Geometry: final body of the model. Coordinates: model frame, mm. Face numbers are marked on the shaded views. A direction names the side the tool comes from. Give positions to 0.01 mm unless a question says otherwise; leave off trailing zeros. Loops run counter-clockwise (first coordinate to the right, second up) from the corner with the lowest first, then second, coordinate; pieces in that order, holes last. Notation, with made-up numbers: (-14.5, 24.5) -> (-6.5, 24.5) arc R3 cw to (-6.5, 28.5) -> close; hole circle Ø5 at (35.5, 80). An arc over 180 degrees is marked (long way). One line per question, with ' | ' between items. Start each with the question number.
Item 1: Section A-A on y = 12.75. Return loops of the section in (x, z).
Item 2: Section B-B on x = -1.3. Return loops of the section in (y, z).
Item 3: Set-up query: the marked faces 1, 2 and 3. Return all of +Z, -Z, +X, -X, +Y, -Y with unobstructed straight access to the full face (end or side cutting, diameter ignored); none if empty.
Item 4: Section D-D on y = 7.25. Return loops of the section in (x, z), then the cut area to 3 significant figures.
Item 5: Mould query, pull axis Z, two halves, no side actions, for the marked faces 4, 5, 6 and 7. Classes: released by +Z, released by -Z, zero draft, split by the parting line, or undercut.
Item 6: Pin query (flat end, axial travel): P1, Ø1.8, axis at x = -0.5, z = 3.5, coming from the -Y side; P2, Ø1.2, axis at y = 4, z = 0, coming from the -X side; P3, Ø3, axis at y = 3.5, z = 1, coming from the +X side. Return the tip coordinate at first contact, or that it passes through.
Item 7: Material intervals for line 1 along Z through (x, y) = (-0.15, 14.5); line 2 along Y through (x, z) = (-2.3, -1.25); line 3 along Z through (x, y) = (-2.05, 13.25), sorted ascending. Write a range as [from, to].
Item 8: Section C-C on z = -0.5. Return loops of the section in (x, y), then the cut area to 3 significant figures.
from build123d import *

# Parameters (mm, degrees)
SKETCH1_W           = 1.506666666
SKETCH1_H           = 1.506666666
BOSS_EXTRUDE1_DEPTH = 15
SKETCH2_R           = 0.753333333
BOSS_EXTRUDE2_DEPTH = 1.666666667
SKETCH3_W           = 5.16
SKETCH3_H           = 1.666666667
SKETCH3_H_2         = 5.16
SKETCH3_W_2         = 1.506666666
SKETCH3_H_3         = 1.506666666
BOSS_EXTRUDE3_DEPTH = 2.5
SKETCH3_3_W         = 5.16
SKETCH3_3_H         = 1.666666667
BOSS_EXTRUDE4_DEPTH = 2.5


with BuildPart() as part:
    # Sketch1 → Boss-Extrude1 (new body)
    with BuildSketch(Plane(origin=(0, 0, 0), x_dir=(1, 0, 0), z_dir=(0, 1, 0))):
        Rectangle(SKETCH1_W, SKETCH1_H)
    extrude(amount=BOSS_EXTRUDE1_DEPTH)

    # Sketch2 → Boss-Extrude2 (add)
    with BuildSketch(Plane.XZ):
        with Locations(Location((0, 0, 0), (0, 0, 270))):
            Circle(SKETCH2_R)
    extrude(amount=BOSS_EXTRUDE2_DEPTH)

    # Sketch3 → Boss-Extrude3 (add)
    # profile 1 of 4: a face of its own
    with BuildSketch(Plane(origin=(0, 15, 0), x_dir=(1, 0, 0), z_dir=(0, 1, 0))):
        with Locations((0, 3.413333334)):
            Rectangle(SKETCH3_W, SKETCH3_H)
    # profile 2 of 4: a face of its own
    with BuildSketch(Plane(origin=(0, 15, 0), x_dir=(1, 0, 0), z_dir=(0, 1, 0))):
        Rectangle(SKETCH3_W, SKETCH3_H_2)
        Rectangle(SKETCH3_W_2, SKETCH3_H_3, mode=Mode.SUBTRACT)
    # profile 3 of 4: a face of its own
    with BuildSketch(Plane(origin=(0, 15, 0), x_dir=(1, 0, 0), z_dir=(0, 1, 0))):
        with Locations((0, -3.413333334)):
            Rectangle(SKETCH3_W, SKETCH3_H)
    # profile 4 of 4: a face of its own
    with BuildSketch(Plane(origin=(0, 15, 0), x_dir=(1, 0, 0), z_dir=(0, 1, 0))):
        Rectangle(SKETCH3_W_2, SKETCH3_H_3)
    extrude(amount=BOSS_EXTRUDE3_DEPTH)

    # Sketch3_3 → Boss-Extrude4 (add)
    with BuildSketch(Plane(origin=(0, 15, 0), x_dir=(1, 0, 0), z_dir=(0, 1, 0))):
        with Locations((0, 3.413333334)):
            Rectangle(SKETCH3_3_W, SKETCH3_3_H)
        with Locations((0, -3.413333334)):
            Rectangle(SKETCH3_3_W, SKETCH3_3_H)
    extrude(amount=-BOSS_EXTRUDE4_DEPTH)


solid = part.part
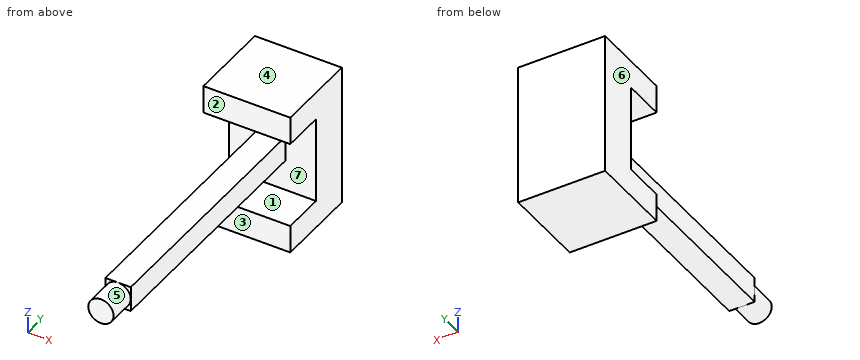
Result sheet:
1) outline: (-2.58, -4.25) -> (2.58, -4.25) -> (2.58, -2.58) -> (-2.58, -2.58) -> close; (-2.58, 2.58) -> (2.58, 2.58) -> (2.58, 4.25) -> (-2.58, 4.25) -> close; (-0.75, -0.75) -> (0.75, -0.75) -> (0.75, 0.75) -> (-0.75, 0.75) -> close
2) outline: (12.5, -4.25) -> (17.5, -4.25) -> (17.5, 4.25) -> (12.5, 4.25) -> (12.5, 2.58) -> (15, 2.58) -> (15, -2.58) -> (12.5, -2.58) -> close
3) face 1: +X, -X, -Y | face 2: +Z, +X, -X, -Y | face 3: -Z, +X, -X, -Y
4) outline: (-0.75, -0.75) -> (0.75, -0.75) -> (0.75, 0.75) -> (-0.75, 0.75) -> close | area: 2.27 mm²
5) face 4: released by +Z | face 5: split by the parting line | face 6: zero draft | face 7: undercut
6) P1: stops at y = 12.5 | P2: stops at x = -0.75 | P3: stops at x = 0.75
7) line 1: z = [-4.25, -2.58], [-0.75, 0.75], [2.58, 4.25] | line 2: y = [15, 17.5] | line 3: z = [-4.25, -2.58], [2.58, 4.25]
8) outline: (-2.58, 15) -> (-0.75, 15) -> (-0.75, 0) -> (-0.56, 0) -> (-0.56, -1.67) -> (0.56, -1.67) -> (0.56, 0) -> (0.75, 0) -> (0.75, 15) -> (2.58, 15) -> (2.58, 17.5) -> (-2.58, 17.5) -> close | area: 37.4 mm²
